```python
from build123d import *

# Parameters (mm, degrees)
F2_T     = -2.5
F3_R     = 2.6
F4_DEPTH = 4


with BuildPart() as f1:
    # F0 (on Front) → F1 (revolve)
    with BuildSketch(Plane.XZ):
        with BuildLine():
            Line((0, -36.8440513045), (0, -11.8440513045))
            ThreePointArc((0, -11.8440513045), (-2.6878763637, -12.1364585585), (-5.25, -13))
            ThreePointArc((-5.25, -13), (-12.207592746, -27.0319276683), (0, -36.8440513045))
        make_face()
        with BuildLine():
            Line((0, -11.8440513045), (0, -5))
            Line((0, -5), (-6.9, -5))
            add(Edge.make_bspline(
                [(-5.25, -13), (-2.8193239395, -11.8750888924), (-0.9143215768, -7.7015358731), (-6.9, -5)],
                knots=[0, 0, 0, 0, 8.1683841731, 8.1683841731, 8.1683841731, 8.1683841731], degree=3))
            ThreePointArc((-5.25, -13), (-2.6878763637, -12.1364585585), (0, -11.8440513045))
        make_face()
    revolve(axis=Axis((0, 0, -18.4220256523), (0, 0, -1)))

    # F2 (hollow: no face is removed)
    offset(amount=F2_T, kind=Kind.INTERSECTION, mode=Mode.SUBTRACT)

    # F3 (on face) → F4 (join)
    with BuildSketch(Plane.XY.offset(-5)):
        with BuildLine():
            Line((-32, -15), (12, -15))
            ThreePointArc((12, -15), (14.1213203436, -14.1213203436), (15, -12))
            Line((15, -12), (15, 12))
            ThreePointArc((15, 12), (14.1213203436, 14.1213203436), (12, 15))
            Line((12, 15), (-32, 15))
            ThreePointArc((-32, 15), (-34.1213203436, 14.1213203436), (-35, 12))
            Line((-35, 12), (-35, -12))
            ThreePointArc((-35, -12), (-34.1213203436, -14.1213203436), (-32, -15))
        make_face()
        with Locations((-20, 0)):
            Circle(F3_R, mode=Mode.SUBTRACT)
    extrude(amount=F4_DEPTH)


solid = f1.part
```
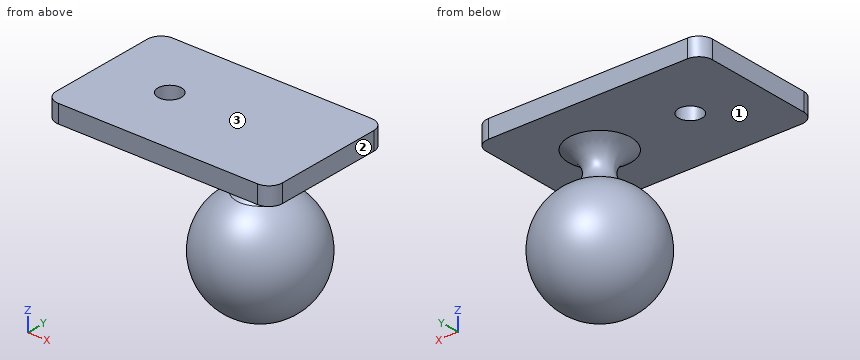
For this review, take the finished solid that the model builds, in its own axes (mm). Face numbers are marked on the shaded views. Round coordinates to 2 decimals unless told otherwise and drop trailing zeros. Order: outer loops, then holes, each group sorted by start corner. A loop starts at its lowest first (then second) coordinate and runs counter-clockwise, first axis right, second up.
Q1. We need section C-C, the plane x = -9. Give the boundary of the cut face in (y, z), plus the area to 3 significant figures.
Findings below:
outline: (-15, -5) - (15, -5) - (15, -1) - (-15, -1) - close; circle Ø17.35 at (0, -24.34); hole circle Ø8.72 at (0, -24.34)
area: 297 mm2
Q2. We need section A-A, the plane x = -20. Give the boundary of the cut face in (y, z), plus the area to 3 significant figures.
Findings below:
outline: (-15, -5) - (-2.6, -5) - (-2.6, -1) - (-15, -1) - close; (2.6, -5) - (15, -5) - (15, -1) - (2.6, -1) - close
area: 99.2 mm2
Q3. We need section B-B, the plane y = 0. State how many separate pieces and enclosed holes the cut face has, plus the area to 3 significant figures.
Findings below:
separate pieces: 2
enclosed holes: 1
area: 396 mm2
Q4. Insertion check: P1, Ø6, axis at x = -24.5, y = -10, coming from the -Z side; P2, Ø6, axis at x = 0, z = -13, coming from the +Y side; P3, Ø8, axis at x = 3, y = -6, coming from the -Z side; P4, Ø2, axis at x = -14, z = -7, coming from the +Y side. Each pin has a flat end and moves straight along its axis. Give the tip position at first contact, or say it passes through.
Findings below:
P1: stops at z = -5
P2: stops at y = 9.31
P3: stops at z = -36.55
P4: passes through
Q5. Wall thickness on line 1 (Z direction, x = -4, y = 7.5); line 2 (Y direction, x = -20, z = -2.85); line 3 (Z direction, x = 2.5, y = -7.5): over which ranges is each line inside the solid? List them lowest first.
Findings below:
line 1: z = -33.51 to -29.61, -19.08 to -15.18, -5 to -1
line 2: y = -15 to -2.6, 2.6 to 15
line 3: z = -34.03 to -30.47, -18.22 to -14.66, -5 to -1
Q6. Mouldability with a two-part tool opening along Z and no side actions: class the marked faces 1, 2 and 3 as pulls with the +Z half, pulls with the -Z half, needs draft (parallel to the pull), parting line crosses it, or undercut.
Findings below:
face 1: undercut
face 2: needs draft
face 3: pulls with the +Z half
Q7. We need section D-D, the plane z = -24.5. Give the boundary of the cut face in (x, y).
Findings below:
outline: circle Ø25 at (0, 0); hole circle Ø20 at (0, 0)
